The drawing under review shows one solid part. Ordinate dimensions are in mm from its lowest x, y, z. Give positions to 0.01 mm unless a question says otherwise; leave off trailing zeros. Write each loop counter-clockwise with the first axis right and the second up, starting at its lowest first coordinate (ties: lowest second). Pieces come first, ordered by that corner, then holes. Notation, with made-up numbers: (76.25, 41.5) - (115.25, 41.5) arc R8 cw to (115.25, 50.5) - close; hole circle Ø9 at (32, -13.75). An arc over 180 degrees is marked (long way). Write each question's results on one line, items separated by ' | '. Start each with the question number.
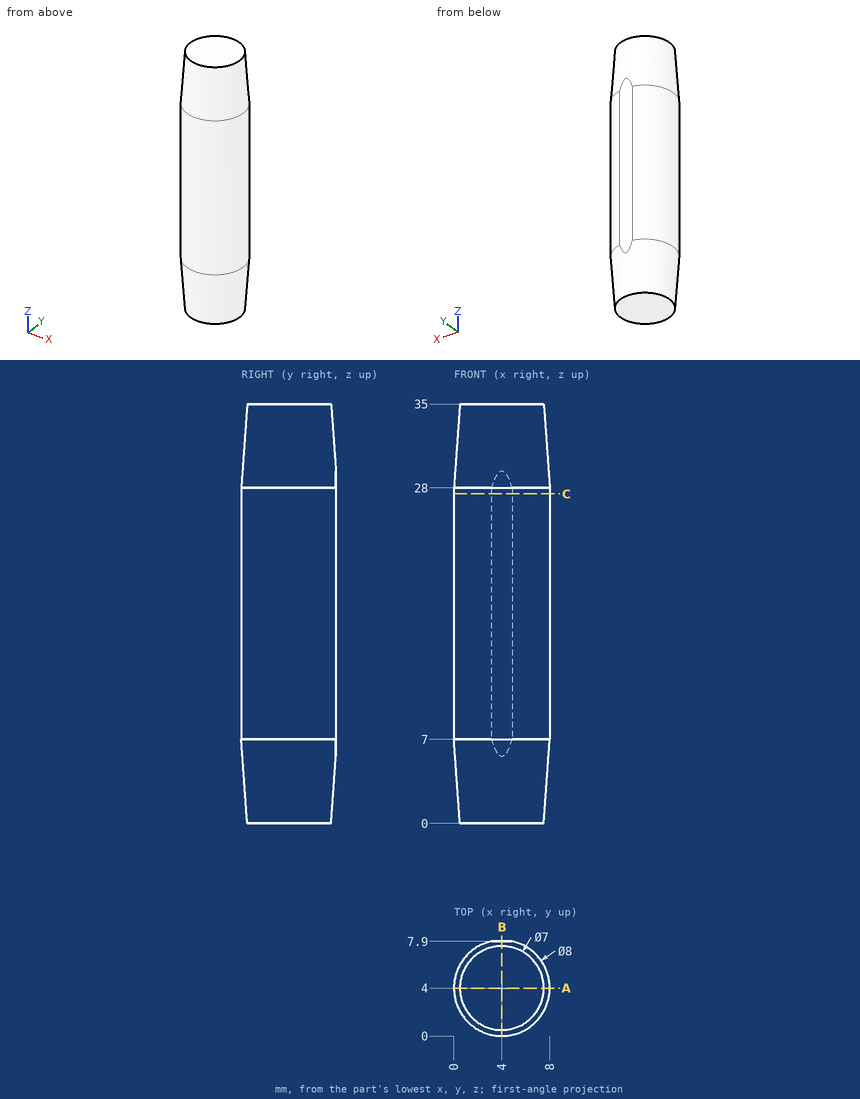
Q1. Add section B-B on x = 4. State the section outline as (y, z) points.
Q2. Add section A-A on y = 4. State the section outline as (x, z) points.
Q3. Add section C-C on z = 27.5. State the section outline as (x, y) points, plus the area to 3 significant figures.
Q4. For line 1 along X through (y, z) = (4.25, 25.5); line 2 along Y through (x, z) = (5, 4); line 3 along X through (y, z) = (5, 10), list the stretches that pass through material, from the lowest coordinate up. Write a range as [from, to].
Result:
1) outline: (0, 7) - (0.5, 0) - (7.5, 0) - (7.9, 5.6) - (7.9, 29.4) - (7.5, 35) - (0.5, 35) - (0, 28) - close
2) outline: (0, 7) - (0.5, 0) - (7.5, 0) - (8, 7) - (8, 28) - (7.5, 35) - (0.5, 35) - (0, 28) - close
3) outline: (3.11, 7.9) arc R4 ccw (long way) to (4.89, 7.9) - close | area: 50.1 mm²
4) line 1: x = [0.01, 7.99] | line 2: y = [0.35, 7.65] | line 3: x = [0.13, 7.87]
